from build123d import *

# Parameters (mm, degrees)
F1_DEPTH = 10


# Not quite as in the source:
# - a feature names something its author has since deleted; it is built from what else it names


with BuildPart() as f1:
    # F0 (on Top) → F1 (new body)
    with BuildSketch(Plane.XY):
        with BuildLine():
            ThreePointArc((2.3611111111, 0.8216777477), (0, -2.5), (-2.3611111111, 0.8216777477))
            ThreePointArc((-2.3611111111, 0.8216777477), (-2.25, 1.4790199458), (-2.3611111111, 2.1363621439))
            ThreePointArc((-2.3611111111, 2.1363621439), (-2.4106719576, 2.2957252286), (-2.4494897428, 2.4580398915))
            Line((-2.4494897428, 2.4580398915), (-2.9577320216, 2.9439046938))
            ThreePointArc((-2.9577320216, 2.9439046938), (-3.1792292558, 2.9811663012), (-3.2956726945, 2.7890976215))
            ThreePointArc((-3.2956726945, 2.7890976215), (-3.2386938705, 2.3249032452), (-3.1166666667, 1.8734252646))
            ThreePointArc((-3.1166666667, 1.8734252646), (-3.05, 1.4790199458), (-3.1166666667, 1.0846146269))
            ThreePointArc((-3.1166666667, 1.0846146269), (0, -3.3), (3.1166666667, 1.0846146269))
            ThreePointArc((3.1166666667, 1.0846146269), (3.05, 1.4790199458), (3.1166666667, 1.8734252646))
            ThreePointArc((3.1166666667, 1.8734252646), (3.2386938705, 2.3249032452), (3.2956726945, 2.7890976215))
            ThreePointArc((3.2956726945, 2.7890976215), (3.1792292558, 2.9811663012), (2.9577320216, 2.9439046938))
            Line((2.9577320216, 2.9439046938), (2.4494897428, 2.4580398915))
            ThreePointArc((2.4494897428, 2.4580398915), (2.4106719576, 2.2957252286), (2.3611111111, 2.1363621439))
            ThreePointArc((2.3611111111, 2.1363621439), (2.25, 1.4790199458), (2.3611111111, 0.8216777477))
        make_face()
    extrude(amount=F1_DEPTH)


solid = f1.part
Work out the finished part from the listing and answer in its coordinate system (mm). A direction names the side the tool comes from. Coordinates: 2 decimals unless noted, no trailing zeros. Loops run counter-clockwise (first coordinate to the right, second up) from the corner with the lowest first, then second, coordinate; pieces in that order, holes last. Notation, with made-up numbers: M 75,0.5 L 96,0.5 A10 cw 96,13.5 Z; hole C 77.5,-39.75 d6. An arc over 180 degrees is marked long. Answer in a Markdown table with one row per item. Add a question column.
1. Consider L1, parallel to X at y = 0, z = 8.25; L2, parallel to X at y = -2, z = 5.5; L3, parallel to Y at x = -2.75, z = 8. Determine where each line is inside the solid, lowest interval first.
2. Find section B-B, the plane z = 1.5. Write down the section's boundary in (x, y), then the cut area to 3 significant figures.
3. Flat-ended cylindrical pins translate along their axes: P1, Ø2, axis at x = 1.5, y = 1, coming from the -Z side; P2, Ø1, axis at x = 1, y = 1, coming from the +Z side. Find the tip coordinate at first contact, or state that the pin passes through.
4. Find section A-A, the plane y = 0. Write down the section's boundary in (x, z).
5. The mould has two halves that part along X. Classify faces 5 (the cylindrical face through (-2.25, 1.47, 4.93)), 6 (the cylindrical face through (-0.1, -3.3, 4.9)), 7 (the flat face through (0, -3, 10)): pulls with the +X half, pulls with the -X half, needs draft (parallel to the pull), parting line crosses it, or undercut.
6. Find section D-D, the plane y = 2. Write down the section's boundary in (x, z), then the cut area to 3 significant figures.
7. A tool of negligible diameter and unlimited length cuts with its end or side. For faces 1 (the cylindrical face through (3.237, 2.318, 4.93)), 2 (the flat face through (0, -3, 0)), 3 (the cylindrical face through (2.25, 1.49, 4.93)), 4 (the cylindrical face through (-3.24, 2.33, 4.93)), from which of +Z, -Z, +X, -X, +Y, -Y can it reach the whole face along a straight path? Write none if from no direction.
8. Find section C-C, the plane x = 0. Write down the section's boundary in (y, z).
Reported:
| question | item | result |
|---|---|---|
| 1 | L1 | x = -3.3 to -2.5, 2.5 to 3.3 |
| 1 | L2 | x = -2.62 to -1.5, 1.5 to 2.62 |
| 1 | L3 | y = -1.82 to 2.75 |
| 2 | outline | M -3.3,2.79 A3.3 ccw -3.12,1.87 A1.2 cw -3.12,1.08 A3.3 ccw long 3.12,1.08 A1.2 cw 3.12,1.87 A3.3 ccw 3.3,2.79 A0.2 ccw 2.96,2.94 L 2.45,2.46 A2.5 cw 2.36,2.14 A2 ccw 2.36,0.82 A2.5 cw long -2.36,0.82 A2 ccw -2.36,2.14 A2.5 cw -2.45,2.46 L -2.96,2.94 A0.2 ccw Z |
| 2 | area | 11.9 mm^2 |
| 3 | P1 | stops at z = 0 |
| 3 | P2 | passes through |
| 4 | outline | M -3.3,0 L -2.5,0 L -2.5,10 L -3.3,10 Z; M 2.5,0 L 3.3,0 L 3.3,10 L 2.5,10 Z |
| 5 | face 5 | undercut |
| 5 | face 6 | parting line crosses it |
| 5 | face 7 | needs draft |
| 6 | outline | M -3.16,0 L -2.32,0 L -2.32,10 L -3.16,10 Z; M 2.32,0 L 3.16,0 L 3.16,10 L 2.32,10 Z |
| 6 | area | 16.8 mm^2 |
| 7 | face 1 | +Z, -Z, +X |
| 7 | face 2 | -Z, +X, -X, +Y, -Y |
| 7 | face 3 | +Z, -Z |
| 7 | face 4 | +Z, -Z, -X |
| 8 | outline | M -3.3,0 L -2.5,0 L -2.5,10 L -3.3,10 Z |
